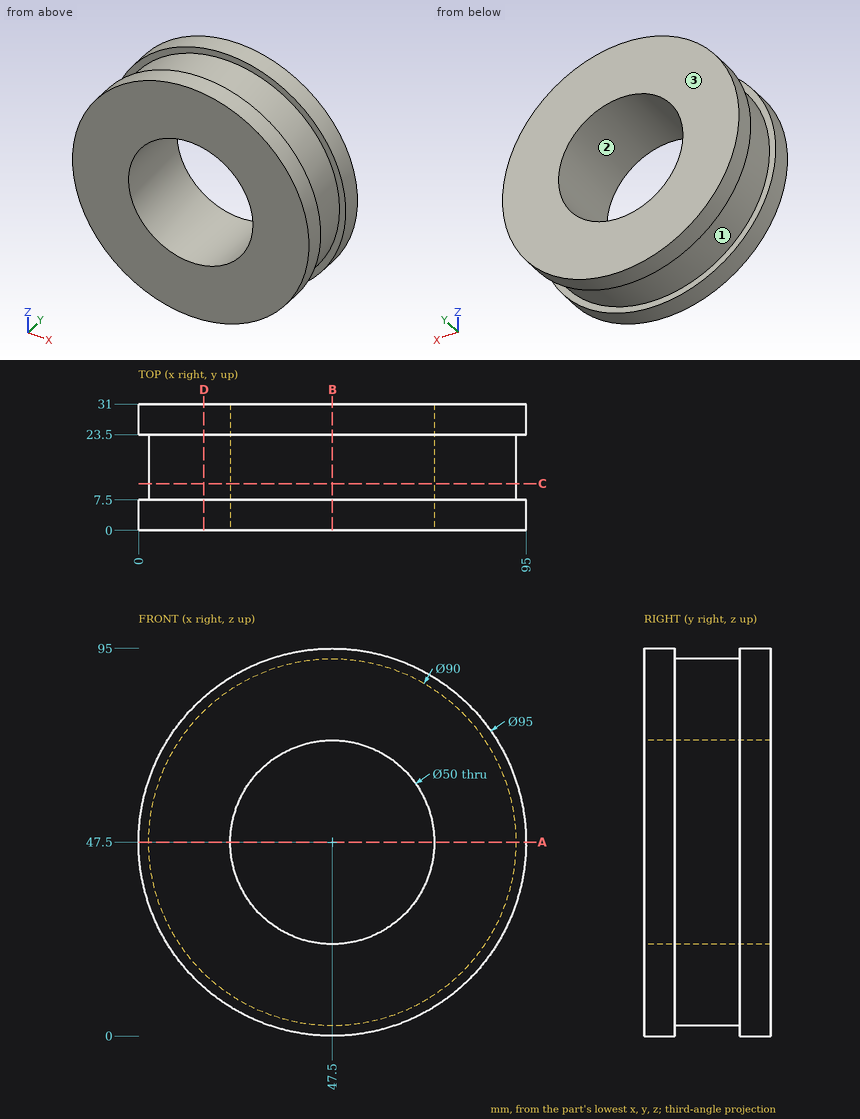
Can you work these out from the drawing? Everything is in mm from the part's minimum corner. Give positions to 0.01 mm unless a question says otherwise; leave off trailing zeros. Loops run counter-clockwise (first coordinate to the right, second up) from the corner with the lowest first, then second, coordinate; pieces in that order, holes last. Notation, with made-up numbers: (-3, -6) -> (13, -6) arc R17 ccw to (13, 27) -> close; hole circle Ø6 at (46, 41). An arc over 180 degrees is marked (long way). Return JSON: item names as keys, results as strings.
Item 1: If we section it at C-C on y = 11.5: List the corners of the cut face in (x, z) for me, plus the area to 3 significant figures.
Geometry results:
{"outline": "circle Ø90 at (47.5, 47.5); hole circle Ø50 at (47.5, 47.5)", "area": "4,400 mm²"}
Item 2: I'm going to push flat-ended pins straight in: pin 1 (1.5 mm diameter, centred on y = 3.5, z = 54, fed in from +X); pin 2 (1.5 mm diameter, centred on y = 14.5, z = 84.5, fed in from -X); pin 3 (2 mm diameter, centred on y = 11, z = 61.5, fed in from -X). Where does each tip first touch, or does it pass through?
Geometry results:
{"pin 1": "stops at x = 94.65", "pin 2": "stops at x = 20.84", "pin 3": "stops at x = 4.42"}
Item 3: If we section it at D-D on x = 16: List the corners of the cut face in (y, z) for me.
Geometry results:
{"outline": "(0, 11.95) -> (7.5, 11.95) -> (7.5, 15.36) -> (23.5, 15.36) -> (23.5, 11.95) -> (31, 11.95) -> (31, 83.05) -> (23.5, 83.05) -> (23.5, 79.64) -> (7.5, 79.64) -> (7.5, 83.05) -> (0, 83.05) -> close"}
Item 4: If we section it at B-B on x = 47.5: List the corners of the cut face in (y, z) for me, plus the area to 4 significant figures.
Geometry results:
{"outline": "(0, 0) -> (7.5, 0) -> (7.5, 2.5) -> (23.5, 2.5) -> (23.5, 0) -> (31, 0) -> (31, 22.5) -> (0, 22.5) -> close; (0, 72.5) -> (31, 72.5) -> (31, 95) -> (23.5, 95) -> (23.5, 92.5) -> (7.5, 92.5) -> (7.5, 95) -> (0, 95) -> close", "area": "1,315 mm²"}
Item 5: If we section it at A-A on z = 47.5: List the corners of the cut face in (x, y) for me.
Geometry results:
{"outline": "(0, 0) -> (22.5, 0) -> (22.5, 31) -> (0, 31) -> (0, 23.5) -> (2.5, 23.5) -> (2.5, 7.5) -> (0, 7.5) -> close; (72.5, 0) -> (95, 0) -> (95, 7.5) -> (92.5, 7.5) -> (92.5, 23.5) -> (95, 23.5) -> (95, 31) -> (72.5, 31) -> close"}
Item 6: I need wall thicknesses on L1, parallel to Z at x = 47, y = 21 (3 decimals); L2, parallel to Y at x = 74.5, z = 85. Which ranges of each line are inside material? Lowest first, please. Write a range as from..to.
Geometry results:
{"L1": "z = 2.503..22.505, 72.495..92.497", "L2": "y = 0..7.5, 23.5..31"}
Item 7: We'd pull the mould along Z, two halves only. Please class the marked faces 1, 2 and 3: +Z half, -Z half, draft (parallel to the pull), parting line (faces both ways), or undercut.
Geometry results:
{"face 1": "parting line", "face 2": "undercut", "face 3": "draft"}
